Read the model definition and answer for the solid it produces. Units are mm, in the model's axes. A direction names the side the tool comes from. Coordinates: 2 decimals unless noted, no trailing zeros. Write each loop counter-clockwise with the first axis right and the second up, starting at its lowest first coordinate (ties: lowest second). Pieces come first, ordered by that corner, then holes.
1) The part is cut by section C-C (x = -128.5). Determine the outline of the cut face in (y, z).
2) Each of these flat-tipped pins is pushed along its axis until it touches: pin 1 Ø10 at (y, z) = (-5.5, 18.5) entering from +X; pin 2 Ø10 at (y, z) = (-0.5, 5.5) entering from +X; pin 3 Ø10 at (y, z) = (-7, -4.5) entering from +X. Where does it stop, or does it pass through?
3) The part is cut by section D-D (x = 20.5). Determine the outline of the cut face in (y, z), then the cut area to 3 significant figures.
4) Determine the mould class of faces 4 (the face through (-254.525, 0.703, 0.42)), 5 (the face through (28.959, -9, -10.3)), 6 (the face through (-93.803, -2.994, 22.804)) for opening direction Y: +Y half, -Y half, draft (parallel to the pull), parting line (faces both ways), or undercut.
5) The part is cut by section A-A (z = 0). Determine the outline of the cut face in (x, y).
6) Which of the six approach directions +Z, -Z, +X, -X, +Y, -Y give full straight-line access (tool end or side, diameter ignored) to faces 1 (the face through (16.959, 9, -10.3)), 2 (the face through (14.001, -13.887, -10.648)), 3 (the face through (-263.541, 0, 0))?
7) Find the intervals of material crossed by line 1 (X direction, y = -21, z = 5); line 2 (X direction, y = 13, z = 15); line 3 (X direction, y = -9, z = 18), in increasing order.
from build123d import *

# Parameters (mm, degrees)
CHAMFER1_SIZE      = 2
SKETCH5_R          = 16
CUT_EXTRUDE2_DEPTH = 61


with BuildPart() as part:
    # Sketch1 → Revolve1 (revolve)
    with BuildSketch(Plane.XY):
        with BuildLine():
            Line((-263.540634281, 0), (-263.540634281, 30))
            Line((-263.540634281, 30), (-213.540634281, 30))
            Line((-213.540634281, 30), (-213.540634281, 17.5))
            Line((-213.540634281, 17.5), (-201.540634281, 17.5))
            Line((-201.540634281, 17.5), (-201.540634281, 23))
            Line((-201.540634281, 23), (10.959365719, 23))
            Line((10.959365719, 23), (10.959365719, 17.5))
            Line((10.959365719, 17.5), (16.959365719, 17.5))
            Line((16.959365719, 17.5), (16.959365719, 13.5))
            Line((16.959365719, 13.5), (28.959365719, 13.5))
            Line((28.959365719, 13.5), (28.959365719, 17.5))
            ThreePointArc((28.959365719, 17.5), (41.333734389, 12.374368671), (46.459365719, 0))
            Line((46.459365719, 0), (-263.540634281, 0))
        make_face()
    revolve(axis=Axis((-145.227257267, 0, 0), (1, 0, 0)))

    # Chamfer1
    chamfer1_edges = [part.edges().sort_by_distance(p)[0] for p in [
        (-213.540634281, -30, 0),
        (-263.540634281, -30, 0),
    ]]
    chamfer(chamfer1_edges, length=CHAMFER1_SIZE)

    # Sketch5 → Cut-Extrude2 (cut, through all)
    with BuildSketch(Plane.XY.offset(30)):
        with Locations((-238.540634281, 0)):
            Circle(SKETCH5_R)
    extrude(amount=-CUT_EXTRUDE2_DEPTH, mode=Mode.SUBTRACT)


solid = part.part
Reported:
1. outline: circle Ø46 at (0, 0)
2. pin 1: stops at x = 39.05
2. pin 2: stops at x = 46.45
2. pin 3: stops at x = 46.14
3. outline: circle Ø27 at (0, 0)
3. area: 573 mm2
4. face 4: undercut
4. face 5: draft
4. face 6: parting line
5. outline: (-263.54, -28) - (-261.54, -30) - (-215.54, -30) - (-213.54, -28) - (-213.54, -17.5) - (-201.54, -17.5) - (-201.54, -23) - (10.96, -23) - (10.96, -17.5) - (16.96, -17.5) - (16.96, -13.5) - (28.96, -13.5) - (28.96, -17.5) arc R17.5 ccw to (28.96, 17.5) - (28.96, 13.5) - (16.96, 13.5) - (16.96, 17.5) - (10.96, 17.5) - (10.96, 23) - (-201.54, 23) - (-201.54, 17.5) - (-213.54, 17.5) - (-213.54, 28) - (-215.54, 30) - (-261.54, 30) - (-263.54, 28) - close; hole circle Ø32 at (-238.54, 0)
6. face 1: none
6. face 2: +X
6. face 3: +Z, -Z, -X, +Y, -Y
7. line 1: x = -263.54 to -213.54, -201.54 to 10.96
7. line 2: x = -263.54 to -247.87, -229.21 to -213.54, -201.54 to 10.96
7. line 3: x = -263.54 to -251.77, -225.31 to -213.54, -201.54 to 10.96
